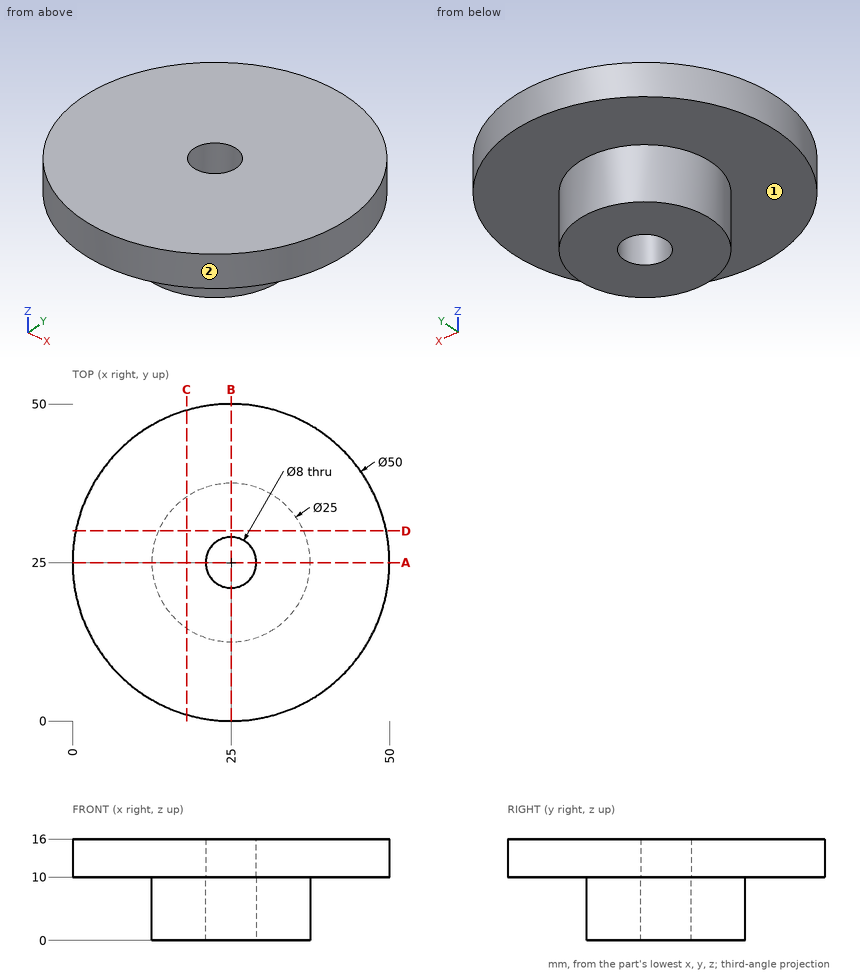
Check sheet for the drawn part. Datum: minimum x, y, z corner. Units: mm. A direction names the side the tool comes from. Give positions to 0.01 mm unless a question says otherwise; leave off trailing zeros. Order: outer loops, then holes, each group sorted by start corner. A loop starts at its lowest first (then second) coordinate and runs counter-clockwise, first axis right, second up. Notation, with made-up numbers: (87, 51) - (134, 51) arc R26 ccw to (134, 90) - close; hole circle Ø8 at (37.5, 48.25). An arc over 180 degrees is marked (long way). Answer in a Markdown table with one row per item. Add a question column.
Q1. Gauge pin test, flat ends, axial feed: pin 1 (12 mm diameter, centred on x = 24, y = 18, fed in from -Z); pin 2 (2 mm diameter, centred on x = 27.5, z = 11.5, fed in from +Y); pin 3 (1 mm diameter, centred on x = 39, z = 11.5, fed in from -Y); pin 4 (8 mm diameter, centred on x = 15, y = 7, fed in from -Z). Record the tip position at first contact, or that the pin passes through.
Q2. Cross-section at C-C, the plane x = 18. Enter the section's corners in (y, z).
Q3. Tool access check on the marked faces 1 and 2. Record the directions out of +Z, -Z, +X, -X, +Y, -Y that give a thin tool (end or side, any length) a straight path to the whole face; none if there is none.
Q4. Cross-section at A-A, the plane y = 25. Enter the section's corners in (x, z).
Q5. Cross-section at D-D, the plane y = 30. Enter the section's corners in (x, z).
Q6. Material ranges on probe 1 along Y at (x, z) = (25, 5); probe 2 along Y at (x, z) = (25, 12.8); probe 3 along Z at (x, y) = (43, 15.5), recorded low to high. Write a range as from..to.
Check values:
| question | item | result |
|---|---|---|
| 1 | pin 1 | stops at z = 0 |
| 1 | pin 2 | stops at y = 49.95 |
| 1 | pin 3 | stops at y = 3.96 |
| 1 | pin 4 | stops at z = 10 |
| 2 | outline | (1, 10) - (14.64, 10) - (14.64, 0) - (35.36, 0) - (35.36, 10) - (49, 10) - (49, 16) - (1, 16) - close |
| 3 | face 1 | -Z |
| 3 | face 2 | +Z, -Z |
| 4 | outline | (0, 10) - (12.5, 10) - (12.5, 0) - (21, 0) - (21, 16) - (0, 16) - close; (29, 0) - (37.5, 0) - (37.5, 10) - (50, 10) - (50, 16) - (29, 16) - close |
| 5 | outline | (0.51, 10) - (13.54, 10) - (13.54, 0) - (36.46, 0) - (36.46, 10) - (49.49, 10) - (49.49, 16) - (0.51, 16) - close |
| 6 | probe 1 | y = 12.5..21, 29..37.5 |
| 6 | probe 2 | y = 0..21, 29..50 |
| 6 | probe 3 | z = 10..16 |
